Check sheet for the modelled part. Datum: model origin and axes. Units: mm. Give positions to 0.01 mm unless a question says otherwise; leave off trailing zeros. Answer as CSV lines item,"result". Start each with the question number.
(1) Material ranges on line 1 (X direction, y = 1.9, z = 76); line 2 (X direction, y = 1.15, z = 46); line 3 (X direction, y = 1.5, z = 67), recorded low to high. Write a range as from..to.
(2) Section check A-A on x = 7. State how many separate pieces and enclosed holes the cut face has, plus the area to 3 significant figures.
(3) Release check for a two-part mould opening along X. For faces 1 (the face through (0, 2, -1)), 2 (the face through (25.75, 1.01, -93.57)), 3 (the face through (-22.218, 0.986, 65.482)), 4 (the face through (-25.82, 1.01, 93.5)) record: pulls with the +X half, pulls with the -X half, needs draft (parallel to the pull), parting line crosses it, or undercut.
from build123d import *

# Parameters (mm, degrees)
SKETCH1_W            = 54.5
SKETCH1_H            = 190
BOSS_EXTRUDE1_DEPTH  = 2
M3_CLEARANCE_HOLE1_D = 3.6
CUT_EXTRUDE1_DEPTH   = 99.851213953
FILLET1_R            = 5


with BuildPart() as part:
    # Sketch1 → Boss-Extrude1 (new body)
    with BuildSketch(Plane(origin=(0, 0, 0), x_dir=(1, 0, 0), z_dir=(0, 1, 0))):
        Rectangle(SKETCH1_W, SKETCH1_H)
    extrude(amount=BOSS_EXTRUDE1_DEPTH)

    # M3 Clearance Hole1 (through all)
    with Locations(Plane(origin=(0, 2, 0), x_dir=(1, 0, 0), z_dir=(0, 1, 0))):
        with Locations((-21.25, 67), (-21.25, 31), (21.25, 67), (21.25, 31), (21.25, -31), (21.25, -67), (-21.25, -67), (-21.25, -31)):
            Hole(M3_CLEARANCE_HOLE1_D / 2)

    # Sketch5 → Cut-Extrude1 (cut, through all)
    with BuildSketch(Plane(origin=(0, 2, 0), x_dir=(1, 0, 0), z_dir=(0, 1, 0))):
        with BuildLine():
            Line((-18.25, 87), (-18.25, 75))
            ThreePointArc((-18.25, 75), (-20.25, 73), (-22.25, 75))
            Line((-22.25, 75), (-22.25, 87))
            ThreePointArc((-22.25, 87), (-20.25, 89), (-18.25, 87))
        make_face()
        with BuildLine():
            Line((18.25, 87), (18.25, 75))
            ThreePointArc((18.25, 75), (20.25, 73), (22.25, 75))
            Line((22.25, 75), (22.25, 87))
            ThreePointArc((22.25, 87), (20.25, 89), (18.25, 87))
        make_face()
        with BuildLine():
            Line((-10, 86.885191349), (10, 86.885191349))
            ThreePointArc((10, 86.885191349), (12, 84.885191349), (10, 82.885191349))
            Line((10, 82.885191349), (-10, 82.885191349))
            ThreePointArc((-10, 82.885191349), (-12, 84.885191349), (-10, 86.885191349))
        make_face()
        with BuildLine():
            Line((-10, 73.885191349), (10, 73.885191349))
            ThreePointArc((10, 73.885191349), (12, 71.885191349), (10, 69.885191349))
            Line((10, 69.885191349), (-10, 69.885191349))
            ThreePointArc((-10, 69.885191349), (-12, 71.885191349), (-10, 73.885191349))
        make_face()
        with BuildLine():
            Line((-10, 60.885191349), (10, 60.885191349))
            ThreePointArc((10, 60.885191349), (12, 58.885191349), (10, 56.885191349))
            Line((10, 56.885191349), (-10, 56.885191349))
            ThreePointArc((-10, 56.885191349), (-12, 58.885191349), (-10, 60.885191349))
        make_face()
        with BuildLine():
            Line((-10, 47.885191349), (10, 47.885191349))
            ThreePointArc((10, 47.885191349), (12, 45.885191349), (10, 43.885191349))
            Line((10, 43.885191349), (-10, 43.885191349))
            ThreePointArc((-10, 43.885191349), (-12, 45.885191349), (-10, 47.885191349))
        make_face()
        with BuildLine():
            Line((-10, 34.885191349), (10, 34.885191349))
            ThreePointArc((10, 34.885191349), (12, 32.885191349), (10, 30.885191349))
            Line((10, 30.885191349), (-10, 30.885191349))
            ThreePointArc((-10, 30.885191349), (-12, 32.885191349), (-10, 34.885191349))
        make_face()
        with BuildLine():
            Line((-10, 21.885191349), (10, 21.885191349))
            ThreePointArc((10, 21.885191349), (12, 19.885191349), (10, 17.885191349))
            Line((10, 17.885191349), (-10, 17.885191349))
            ThreePointArc((-10, 17.885191349), (-12, 19.885191349), (-10, 21.885191349))
        make_face()
        with BuildLine():
            Line((-10, 8.885191349), (10, 8.885191349))
            ThreePointArc((10, 8.885191349), (12, 6.885191349), (10, 4.885191349))
            Line((10, 4.885191349), (-10, 4.885191349))
            ThreePointArc((-10, 4.885191349), (-12, 6.885191349), (-10, 8.885191349))
        make_face()
        with BuildLine():
            Line((-19.25, 57.932734115), (-19.25, 40.067265885))
            ThreePointArc((-19.25, 40.067265885), (-21.25, 38.067265885), (-23.25, 40.067265885))
            Line((-23.25, 40.067265885), (-23.25, 57.932734115))
            ThreePointArc((-23.25, 57.932734115), (-21.25, 59.932734115), (-19.25, 57.932734115))
        make_face()
        with BuildLine():
            Line((-19.25, 22.533690779), (-19.25, 8.466309221))
            ThreePointArc((-19.25, 8.466309221), (-21.25, 6.466309221), (-23.25, 8.466309221))
            Line((-23.25, 8.466309221), (-23.25, 22.533690779))
            ThreePointArc((-23.25, 22.533690779), (-21.25, 24.533690779), (-19.25, 22.533690779))
        make_face()
        with BuildLine():
            Line((19.25, 57.932734115), (19.25, 40.067265885))
            ThreePointArc((19.25, 40.067265885), (21.25, 38.067265885), (23.25, 40.067265885))
            Line((23.25, 40.067265885), (23.25, 57.932734115))
            ThreePointArc((23.25, 57.932734115), (21.25, 59.932734115), (19.25, 57.932734115))
        make_face()
        with BuildLine():
            Line((19.25, 22.533690779), (19.25, 8.466309221))
            ThreePointArc((19.25, 8.466309221), (21.25, 6.466309221), (23.25, 8.466309221))
            Line((23.25, 8.466309221), (23.25, 22.533690779))
            ThreePointArc((23.25, 22.533690779), (21.25, 24.533690779), (19.25, 22.533690779))
        make_face()
        with BuildLine():
            Line((-18.25, -87), (-18.25, -75))
            ThreePointArc((-18.25, -75), (-20.25, -73), (-22.25, -75))
            Line((-22.25, -75), (-22.25, -87))
            ThreePointArc((-22.25, -87), (-20.25, -89), (-18.25, -87))
        make_face()
        with BuildLine():
            Line((18.25, -87), (18.25, -75))
            ThreePointArc((18.25, -75), (20.25, -73), (22.25, -75))
            Line((22.25, -75), (22.25, -87))
            ThreePointArc((22.25, -87), (20.25, -89), (18.25, -87))
        make_face()
        with BuildLine():
            Line((-10, -86.885191349), (10, -86.885191349))
            ThreePointArc((10, -86.885191349), (12, -84.885191349), (10, -82.885191349))
            Line((10, -82.885191349), (-10, -82.885191349))
            ThreePointArc((-10, -82.885191349), (-12, -84.885191349), (-10, -86.885191349))
        make_face()
        with BuildLine():
            Line((-10, -73.885191349), (10, -73.885191349))
            ThreePointArc((10, -73.885191349), (12, -71.885191349), (10, -69.885191349))
            Line((10, -69.885191349), (-10, -69.885191349))
            ThreePointArc((-10, -69.885191349), (-12, -71.885191349), (-10, -73.885191349))
        make_face()
        with BuildLine():
            Line((-10, -60.885191349), (10, -60.885191349))
            ThreePointArc((10, -60.885191349), (12, -58.885191349), (10, -56.885191349))
            Line((10, -56.885191349), (-10, -56.885191349))
            ThreePointArc((-10, -56.885191349), (-12, -58.885191349), (-10, -60.885191349))
        make_face()
        with BuildLine():
            Line((-10, -47.885191349), (10, -47.885191349))
            ThreePointArc((10, -47.885191349), (12, -45.885191349), (10, -43.885191349))
            Line((10, -43.885191349), (-10, -43.885191349))
            ThreePointArc((-10, -43.885191349), (-12, -45.885191349), (-10, -47.885191349))
        make_face()
        with BuildLine():
            Line((-10, -34.885191349), (10, -34.885191349))
            ThreePointArc((10, -34.885191349), (12, -32.885191349), (10, -30.885191349))
            Line((10, -30.885191349), (-10, -30.885191349))
            ThreePointArc((-10, -30.885191349), (-12, -32.885191349), (-10, -34.885191349))
        make_face()
        with BuildLine():
            Line((-10, -21.885191349), (10, -21.885191349))
            ThreePointArc((10, -21.885191349), (12, -19.885191349), (10, -17.885191349))
            Line((10, -17.885191349), (-10, -17.885191349))
            ThreePointArc((-10, -17.885191349), (-12, -19.885191349), (-10, -21.885191349))
        make_face()
        with BuildLine():
            Line((-10, -8.885191349), (10, -8.885191349))
            ThreePointArc((10, -8.885191349), (12, -6.885191349), (10, -4.885191349))
            Line((10, -4.885191349), (-10, -4.885191349))
            ThreePointArc((-10, -4.885191349), (-12, -6.885191349), (-10, -8.885191349))
        make_face()
        with BuildLine():
            Line((-19.25, -57.932734115), (-19.25, -40.067265885))
            ThreePointArc((-19.25, -40.067265885), (-21.25, -38.067265885), (-23.25, -40.067265885))
            Line((-23.25, -40.067265885), (-23.25, -57.932734115))
            ThreePointArc((-23.25, -57.932734115), (-21.25, -59.932734115), (-19.25, -57.932734115))
        make_face()
        with BuildLine():
            Line((-19.25, -22.533690779), (-19.25, -8.466309221))
            ThreePointArc((-19.25, -8.466309221), (-21.25, -6.466309221), (-23.25, -8.466309221))
            Line((-23.25, -8.466309221), (-23.25, -22.533690779))
            ThreePointArc((-23.25, -22.533690779), (-21.25, -24.533690779), (-19.25, -22.533690779))
        make_face()
        with BuildLine():
            Line((19.25, -57.932734115), (19.25, -40.067265885))
            ThreePointArc((19.25, -40.067265885), (21.25, -38.067265885), (23.25, -40.067265885))
            Line((23.25, -40.067265885), (23.25, -57.932734115))
            ThreePointArc((23.25, -57.932734115), (21.25, -59.932734115), (19.25, -57.932734115))
        make_face()
        with BuildLine():
            Line((19.25, -22.533690779), (19.25, -8.466309221))
            ThreePointArc((19.25, -8.466309221), (21.25, -6.466309221), (23.25, -8.466309221))
            Line((23.25, -8.466309221), (23.25, -22.533690779))
            ThreePointArc((23.25, -22.533690779), (21.25, -24.533690779), (19.25, -22.533690779))
        make_face()
    extrude(amount=-CUT_EXTRUDE1_DEPTH, mode=Mode.SUBTRACT)

    # Fillet1
    fillet1_edges = [part.edges().sort_by_distance(p)[0] for p in [
        (27.25, 1, 95),
        (-27.25, 1, 95),
        (-27.25, 1, -95),
        (27.25, 1, -95),
    ]]
    fillet(fillet1_edges, radius=FILLET1_R)


solid = part.part
Working result:
1,line 1,"x = -27.25..-22.25, -18.25..18.25, 22.25..27.25"
1,line 2,"x = -27.25..-23.25, -19.25..-12, 12..19.25, 23.25..27.25"
1,line 3,"x = -27.25..-23.05, -19.45..19.45, 23.05..27.25"
2,separate pieces,"15"
2,enclosed holes,"0"
2,area,"268 mm^2"
3,face 1,"needs draft"
3,face 2,"pulls with the +X half"
3,face 3,"undercut"
3,face 4,"pulls with the -X half"
